Source: CAD feature listing. Evaluate the final solid. Frame: model axes, mm. Give positions to 0.01 mm unless a question says otherwise; leave off trailing zeros. Order: outer loops, then holes, each group sorted by start corner. A loop starts at its lowest first (then second) coordinate and runs counter-clockwise, first axis right, second up. Notation, with made-up numbers: M 65.5,19 L 89.5,19 A23 cw 89.5,33 Z; hole C 57,56.25 d2. An arc over 180 degrees is marked long. Use CSV: the item, a comma, the result in double quotes. Start each with the question number.
1. Section query A-A, the plane z = 92.5. Return the cut outline in (x, y), plus the area to 3 significant figures.
2. Pin query (flat end, axial travel): P1, Ø2, axis at x = 4.5, z = 70.5, coming from the -Y side; P2, Ø3.5, axis at x = 3.175, z = 6.35, coming from the -Y side; P3, Ø1.5, axis at x = 3, y = -4, coming from the -Z side. Return the tip coordinate at first contact, or that it passes through.
3. Line query: line 1 along X through (y, z) = (11.75, 6.35); line 2 along Z through (x, y) = (2.25, 4.5); line 3 along Z through (x, y) = (2.25, 5.5). Output: solid intervals per line, ascending. Write a range as [from, to].
4. Section query B-B, the plane y = 32.5. Return the cut outline in (x, z), plus the area to 3 significant figures.
from build123d import *

# Parameters (mm, degrees)
BOSS_EXTRUDE1_DEPTH   = 6.35
F_4_40_TAPPED_HOLE1_D = 2.2606


with BuildPart() as part:
    # Sketch1 → Boss-Extrude1 (new body)
    with BuildSketch(Plane(origin=(0, 0, 0), x_dir=(0, 0, -1), z_dir=(1, 0, 0))):
        with BuildLine():
            Line((0, 0), (0, 12.7))
            ThreePointArc((0, 12.7), (-58.496284585, 31.463125354), (-114.3, 57.15))
            Line((-114.3, 57.15), (-127, 57.15))
            Line((-127, 57.15), (-34.29, -5.08))
            Line((-34.29, -5.08), (-31.75, -5.08))
            Line((-31.75, -5.08), (-31.75, 0))
            Line((-31.75, 0), (0, 0))
        make_face()
    extrude(amount=BOSS_EXTRUDE1_DEPTH)

    # #4-40 Tapped Hole1 (through all)
    with Locations(Plane(origin=(0, 0, 0), x_dir=(-1, 0, 0), z_dir=(0, -1, 0))):
        with Locations((-3.175, -25.4), (-3.175, -6.35)):
            Hole(F_4_40_TAPPED_HOLE1_D / 2)


solid = part.part
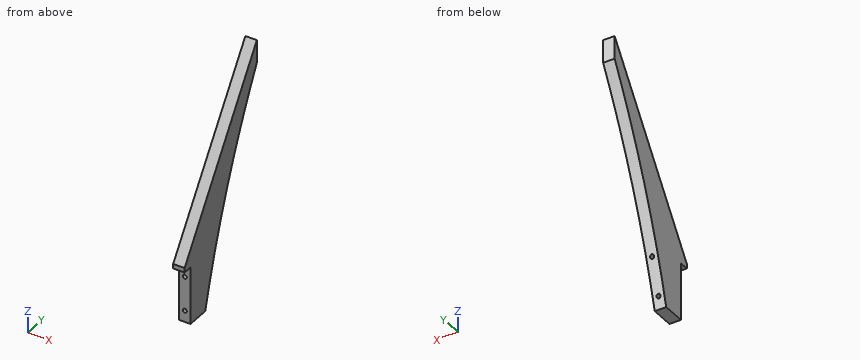
Result set:
1,outline,"M 0,33.99 L 6.35,33.99 L 6.35,46.14 L 0,46.14 Z"
1,area,"77.1 mm2"
2,P1,"y = 18.55"
2,P2,"y = 0"
2,P3,"z = 31.75"
3,line 1,"[0, 2.04], [4.31, 6.35]"
3,line 2,"[0, 5.7], [7, 24.75], [26.05, 48.56]"
3,line 3,"[0, 5.7], [7, 24.75], [26.05, 50.05]"
4,outline,"M 0,61.14 L 6.35,61.14 L 6.35,90.28 L 0,90.28 Z"
4,area,"185 mm2"
